The listing builds one solid part. Answer for the finished solid, in the listing's coordinates (mm). Coordinates: 2 decimals unless noted, no trailing zeros. Loops run counter-clockwise (first coordinate to the right, second up) from the corner with the lowest first, then second, coordinate; pieces in that order, holes last. Notation, with made-up numbers: M 41,80 L 50,80 A30 cw 50,103 Z; hole C 88,35 d5. An arc over 180 degrees is marked long. Return JSON: item names as keys, results as strings. Group by question number.
1. Section D-D (z = 5) is taken. Write down the section's boundary in (x, y).
2. The mould has two halves that part along X. Classify faces 1 (the face through (-37, -10, 17.462)), 2 (the face through (-9.77, 44.01, 17.34)), 3 (the face through (-30.235, 23.183, -0.244)): pulls with the +X half, pulls with the -X half, needs draft (parallel to the pull), parting line crosses it, or undercut.
3. Given P1, Ø4, axis at y = -18.5, z = -10.5, coming from the -X side; P2, Ø3, axis at x = 25, z = -1.5, coming from the +Y side; P3, Ø10, axis at y = -15.5, z = -12.5, coming from the -X side, each flat-ended and moving along its own axis, determine where each tip first touches the part or whether it passes through.
4. Section C-C (z = 13) is taken. Write down the section's boundary in (x, y), then the cut area to 3 significant figures.
5. Straight lines are drawn through the part: L1, parallel to Y at x = -29.5, z = 7; L2, parallel to Y at x = 0, z = -5; L3, parallel to X at y = -9, z = -3.5. For each, find the intervals that lie inside material, in ascending order. Write a range as from..to.
6. Section A-A (x = 0) is taken. Write down the section's boundary in (y, z) (1 decimal), then the cut area to 3 significant figures.
```python
from build123d import *

# Parameters (mm, degrees)
F3_SIZE = 2.032


with BuildPart() as f2:
    # F0 (on Front) → F2 (revolve)
    with BuildSketch(Plane.XZ):
        with BuildLine():
            Line((46.99, 17.4625), (38.1, 17.4625))
            Line((38.1, 17.4625), (38.1, -17.4625))
            Line((38.1, -17.4625), (46.99, -17.4625))
            Line((46.99, -17.4625), (46.99, -9.98304))
            ThreePointArc((46.99, -9.98304), (42.291, 0), (46.99, 9.98304))
            Line((46.99, 9.98304), (46.99, 17.4625))
        make_face()
    revolve(axis=Axis((0, 0, 0.613732), (0, 0, -1)))

    # F3
    f3_edges = [f2.edges().sort_by_distance(p)[0] for p in [
        (-46.99, 0, 17.4625),
        (-46.99, 0, -17.4625),
    ]]
    chamfer(f3_edges, length=F3_SIZE)


solid = f2.part
```
Worked out:
{
 "1": {"outline": "C 0,0 d86.59; hole C 0,0 d76.2"},
 "2": {"face 1": "needs draft", "face 2": "parting line crosses it", "face 3": "undercut"},
 "3": {"P1": "x = -44", "P2": "y = 35.29", "P3": "x = -45.8"},
 "4": {"outline": "C 0,0 d93.98; hole C 0,0 d76.2", "area": "2,380 mm^2"},
 "5": {"L1": "-33.11..-24.11, 24.11..33.11", "L2": "-43.29..-38.1, 38.1..43.29", "L3": "-41.82..-37.02, 37.02..41.82"},
 "6": {"outline": "M -47,-15.4 L -45,-17.5 L -38.1,-17.5 L -38.1,17.5 L -45,17.5 L -47,15.4 L -47,10 A13 cw -47,-10 Z; M 38.1,-17.5 L 45,-17.5 L 47,-15.4 L 47,-10 A13 cw 47,10 L 47,15.4 L 45,17.5 L 38.1,17.5 Z", "area": "482 mm^2"}
}
